Here's how the part is built. I have some questions about the finished solid (model axes, mm). Face numbers are marked on the shaded views. A direction names the side the tool comes from. Round coordinates to 2 decimals unless told otherwise and drop trailing zeros. Order: outer loops, then holes, each group sorted by start corner. A loop starts at its lowest first (then second) coordinate and runs counter-clockwise, first axis right, second up. Notation, with made-up numbers: (88.5, 43.5) -> (105.5, 43.5) arc R19 ccw to (105.5, 60.5) -> close; hole circle Ø2 at (11.25, 16). An arc over 180 degrees is marked (long way). Use a Markdown table: item, result. Add a question column.
(1) I want a section at C-C, the plane y = 10.5. Please give me the cut outline in (x, z) (3 decimals).
(2) If I drill on probe 1 along Z at (x, y) = (-3, 4); probe 2 along Y at (x, z) = (11, 16.5); probe 3 along X at (y, z) = (3, 15.5), over which ranges is the centre line in solid material (lowest first)?
(3) On a 3-axis mill with a long thin cutter (end or side, diameter ignored), from which of +Z, -Z, +X, -X, +Y, -Y can I reach the whole of each face in a straight line? I mean the marked faces 1 and 2. Say none if no direction works.
(4) I want a section at B-B, the plane x = -6. Please give me the cut outline in (y, z).
(5) I want a section at A-A, the plane y = 5.5. Please give me the cut outline in (x, z) (3 decimals), then the cut area to 3 significant figures.
(6) Thinking about a two-plate mould opening in X: for the marked faces 3, 4 and 5, which applies, pulls with the +X half, pulls with the -X half, needs draft (parallel to the pull), parting line crosses it, or undercut?
(7) I want a section at D-D, the plane z = 32.5. Please give me the cut outline in (x, y), then the cut area to 3 significant figures.
(8) I'm going to push flat-ended pins straight in: P1, Ø3, axis at y = 5, z = 40, coming from the -X side; P2, Ø1.9, axis at y = 8, z = 41.5, coming from the +X side (3 decimals); P3, Ø5, axis at x = 0.5, y = 4.5, coming from the +Z side. Where does each tip first touch, or does it pass through?
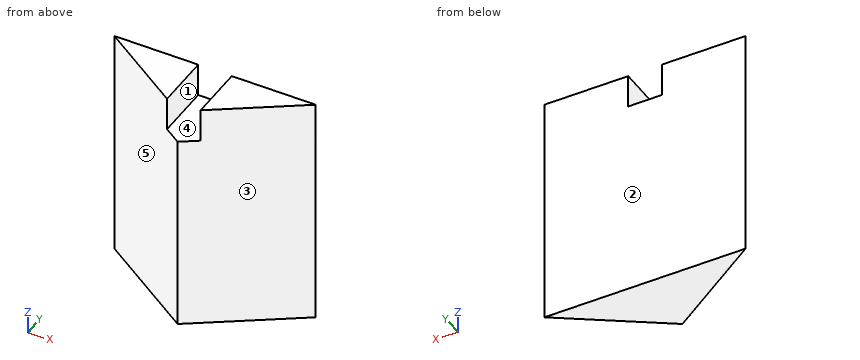
from build123d import *

# Parameters (mm, degrees)
F1_DEPTH = 44.45
F2_W     = 6.35
F2_H     = 6.35
F3_DEPTH = 25.4


with BuildPart() as f1:
    # F0 (on Top) → F1 (new body)
    with BuildSketch(Plane.XY):
        Polygon((-19.05, 12.7), (0, 0), (0, 12.7), (-12.7, 12.7), align=None)
        Polygon((0, 12.7), (0, 0), (19.05, 12.7), (12.7, 12.7), align=None)
    extrude(amount=F1_DEPTH)

    # F2 (on face) → F3 (cut)
    with BuildSketch(Plane(origin=(0, 12.7, 0), x_dir=(-1, 0, 0), z_dir=(0, 1, 0))):
        with Locations((0, 41.275)):
            Rectangle(F2_W, F2_H)
    extrude(amount=-F3_DEPTH, mode=Mode.SUBTRACT)


solid = f1.part
Taken from the geometry:
| question | item | result |
|---|---|---|
| 1 | outline | (-15.75, 0) -> (15.75, 0) -> (15.75, 44.45) -> (3.175, 44.45) -> (3.175, 38.1) -> (-3.175, 38.1) -> (-3.175, 44.45) -> (-15.75, 44.45) -> close |
| 2 | probe 1 | z = 0 to 38.1 |
| 2 | probe 2 | y = 7.33 to 12.7 |
| 2 | probe 3 | x = -4.5 to 4.5 |
| 3 | face 1 | +Z, +Y, -Y |
| 3 | face 2 | +Z, -Z, +X, -X, +Y |
| 4 | outline | (4, 0) -> (12.7, 0) -> (12.7, 44.45) -> (4, 44.45) -> close |
| 5 | outline | (-8.25, 0) -> (8.25, 0) -> (8.25, 44.45) -> (3.175, 44.45) -> (3.175, 38.1) -> (-3.175, 38.1) -> (-3.175, 44.45) -> (-8.25, 44.45) -> close |
| 5 | area | 693 mm2 |
| 6 | face 3 | pulls with the +X half |
| 6 | face 4 | undercut |
| 6 | face 5 | pulls with the -X half |
| 7 | outline | (-19.05, 12.7) -> (0, 0) -> (19.05, 12.7) -> close |
| 7 | area | 242 mm2 |
| 8 | P1 | stops at x = -9.75 |
| 8 | P2 | stops at x = 13.425 |
| 8 | P3 | stops at z = 38.1 |
